Read the model definition and answer for the solid it produces. Units are mm, in the model's axes. Face numbers are marked on the shaded views. Round coordinates to 2 decimals unless told otherwise and drop trailing zeros. Order: outer loops, then holes, each group sorted by start corner. A loop starts at its lowest first (then second) coordinate and runs counter-clockwise, first axis right, second up.
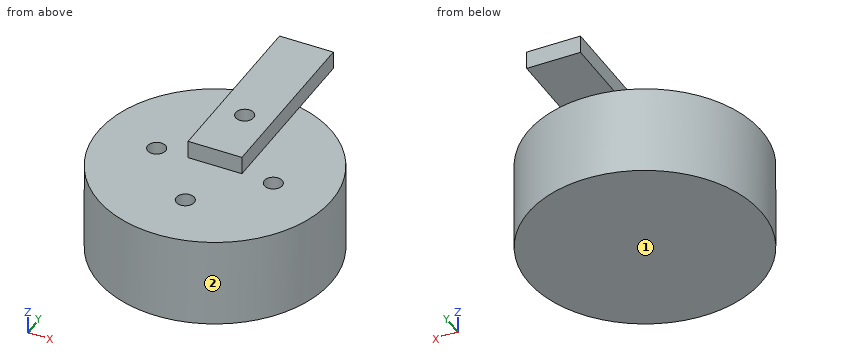
from build123d import *

# Parameters (mm, degrees)
F0_R            = 6.5
F1_DEPTH        = 5
F2_R            = 0.5
F3_DEPTH        = 2
F3_COPIES_COUNT = 4
F4_R            = 0.5
F5_DEPTH        = 1


# Not quite as in the source:
# - a pattern or mirror of a feature is missing from the dataset's text; its kind, count and spacing are read off the source's solid


with BuildPart() as f1:
    # F0 (on Top) → F1 (new body)
    with BuildSketch(Plane.XY):
        Circle(F0_R)
    extrude(amount=F1_DEPTH)

    # F2 (on face) → F3 (cut)
    with BuildSketch(Plane.XY.offset(5)):
        with Locations((0, 3.25)):
            Circle(F2_R)
    f3 = extrude(amount=-F3_DEPTH, mode=Mode.SUBTRACT)

    # F3_copies: F3 ×4 about axis
    f3_copies_axis = Axis((0, 0, 0), (0, 0, 1))
    for i in range(1, F3_COPIES_COUNT):
        add(f3.rotate(f3_copies_axis, i * 360 / F3_COPIES_COUNT), mode=Mode.SUBTRACT)

    # F4 (on face) → F5 (join)
    with BuildSketch(Plane.XY.offset(5)):
        with BuildLine():
            Line((-1.5, 10), (-1.5, 6.3245553203))
            ThreePointArc((-1.5, 6.3245553203), (0, 6.5), (1.5, 6.3245553203))
            Line((1.5, 6.3245553203), (1.5, 10))
            Line((1.5, 10), (-1.5, 10))
        make_face()
        with BuildLine():
            Line((-1.5, 6.3245553203), (-1.5, 0))
            Line((-1.5, 0), (1.5, 0))
            Line((1.5, 0), (1.5, 6.3245553203))
            ThreePointArc((1.5, 6.3245553203), (0, 6.5), (-1.5, 6.3245553203))
        make_face()
        with Locations((0, 3.25)):
            Circle(F4_R, mode=Mode.SUBTRACT)
    extrude(amount=F5_DEPTH)


solid = f1.part
Q1. Flat-ended cylindrical pins translate along their axes: pin 1 (3 mm diameter, centred on x = -4, z = 5.5, fed in from -Y); pin 2 (3.5 mm diameter, centred on x = 0.5, y = 8.5, fed in from -Z); pin 3 (5 mm diameter, centred on x = 0, y = -3.5, fed in from +Z). Find the tip coordinate at first contact, or state that the pin passes through.
Outcome:
pin 1: stops at y = -5.96
pin 2: stops at z = 5
pin 3: stops at z = 5
Q2. For a pull along Y with two mould halves and no side action, classify the marked faces 1 and 2 as released by +Y, released by -Y, zero draft, split by the parting line, or undercut.
Outcome:
face 1: zero draft
face 2: split by the parting line
Q3. A cutting plane is placed at C-C, the plane y = 3.25. Give the vertices of the cut face in (x, z), plus the area to 3 significant figures.
Outcome:
outline: (-5.63, 0) - (5.63, 0) - (5.63, 5) - (1.5, 5) - (1.5, 6) - (0.5, 6) - (0.5, 3) - (-0.5, 3) - (-0.5, 6) - (-1.5, 6) - (-1.5, 5) - (-5.63, 5) - close
area: 56.3 mm2
Q4. A cutting plane is placed at D-D, the plane z = 1.2. Give the vertices of the cut face in (x, y), plus the area to 3 significant figures.
Outcome:
outline: circle Ø13 at (0, 0)
area: 133 mm2
Q5. A cutting plane is placed at A-A, the plane z = 3.2. Give the vertices of the cut face in (x, y), plus the area to 3 significant figures.
Outcome:
outline: circle Ø13 at (0, 0); hole circle Ø1 at (-3.25, 0); hole circle Ø1 at (0, -3.25); hole circle Ø1 at (0, 3.25); hole circle Ø1 at (3.25, 0)
area: 130 mm2
Q6. A cutting plane is placed at B-B, the plane x = 0. Give the vertices of the cut face in (y, z), plus the area to 3 significant figures.
Outcome:
outline: (-6.5, 0) - (6.5, 0) - (6.5, 5) - (10, 5) - (10, 6) - (3.75, 6) - (3.75, 3) - (2.75, 3) - (2.75, 6) - (0, 6) - (0, 5) - (-2.75, 5) - (-2.75, 3) - (-3.75, 3) - (-3.75, 5) - (-6.5, 5) - close
area: 70.0 mm2
Q7. Straight lines are drawn through the part: probe 1 along Y at (x, z) = (0, 3.5); probe 2 along Z at (x, y) = (-4, -0.25); probe 3 along X at (y, z) = (4.25, 5.05). For each, find the intervals that lie inside material, in ascending order.
Outcome:
probe 1: y = -6.5 to -3.75, -2.75 to 2.75, 3.75 to 6.5
probe 2: z = 0 to 5
probe 3: x = -1.5 to 1.5
